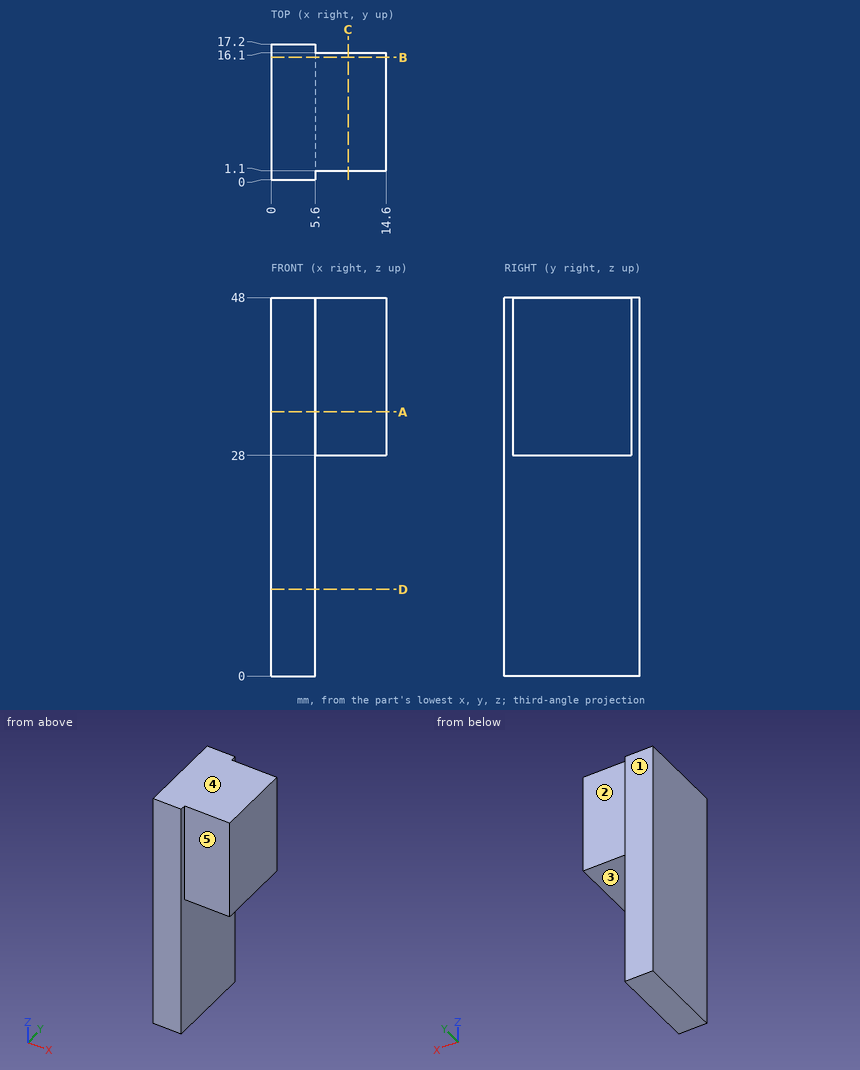
Input: dimensioned drawing with shaded views. Units: mm. Origin: part minimum x, y, z. A direction names the side the tool comes from. Round coordinates to 2 decimals unless told otherwise and drop trailing zeros. Write each loop counter-clockwise with the first axis right and the second up, starting at its lowest first coordinate (ties: lowest second). Pieces come first, ordered by that corner, then holes. Notation, with made-up numbers: (-16.5, 51.5) -> (-8.5, 51.5) arc R20 cw to (-8.5, 70.5) -> close; hole circle Ø5 at (-36.75, 58.5). An arc over 180 degrees is marked (long way). Use CSV: the item, a comma, the result in double quotes. Start each with the question number.
Q1. Section A-A (z = 33.5). Return loops of the section in (x, y).
Q2. Reachability of the marked faces 1, 2, 3, 4 and 5 from +Z, -Z, +X, -X, +Y, -Y: full face, straight path, thin tool, end or side. Return the list, or none.
Q3. Section D-D (z = 11). Return loops of the section in (x, y).
Q4. Section C-C (x = 9.75). Return loops of the section in (y, z), plus the area to 3 significant figures.
Q5. First-contact query: pin 1 Ø7 at (x, y) = (11.5, 12) entering from -Z; pin 2 Ø1.5 at (x, z) = (8.5, 42.5) entering from +Y; pin 3 Ø3 at (y, z) = (12.5, 21) entering from +X. Flat tips, straight axial feed; report the tip coordinate or a pass-through.
Q6. Section B-B (y = 15.5). Return loops of the section in (x, z), plus the area to 3 significant figures.
Q7. Line query: L1, parallel to Y at x = 9, z = 40; L2, parallel to Z at x = 13.25, y = 12.5; L3, parallel to X at y = 13.5, z = 4. Output: solid intervals per line, ascending.
Result sheet:
1,outline,"(0, 0) -> (5.6, 0) -> (5.6, 1.1) -> (14.6, 1.1) -> (14.6, 16.1) -> (5.6, 16.1) -> (5.6, 17.2) -> (0, 17.2) -> close"
2,face 1,"+Z, -Z, +X, -X, +Y"
2,face 2,"+Z, -Z, +X, +Y"
2,face 3,"-Z, +X, +Y, -Y"
2,face 4,"+Z, +X, -X, +Y, -Y"
2,face 5,"+Z, -Z, +X, -Y"
3,outline,"(0, 0) -> (5.6, 0) -> (5.6, 17.2) -> (0, 17.2) -> close"
4,outline,"(1.1, 28) -> (16.1, 28) -> (16.1, 48) -> (1.1, 48) -> close"
4,area,"300 mm²"
5,pin 1,"z = 28"
5,pin 2,"y = 16.1"
5,pin 3,"x = 5.6"
6,outline,"(0, 0) -> (5.6, 0) -> (5.6, 28) -> (14.6, 28) -> (14.6, 48) -> (0, 48) -> close"
6,area,"449 mm²"
7,L1,"1.1 to 16.1"
7,L2,"28 to 48"
7,L3,"0 to 5.6"
